The listing builds one solid part. Answer for the finished solid, in the listing's coordinates (mm). Round coordinates to 2 decimals unless told otherwise and drop trailing zeros. Write each loop counter-clockwise with the first axis right and the second up, starting at its lowest first coordinate (ties: lowest second). Pieces come first, ordered by that corner, then holes.
(1) Find the intervals of material crossed by probe 1 along Z at (x, y) = (25, 0.9); probe 2 along X at (y, z) = (1.8, -12.7); probe 3 along X at (y, z) = (0.45, -62), in increasing order.
(2) A cutting plane is placed at A-A, the plane z = -88.9. Give the vertices of the cut face in (x, y) (3 decimals).
(3) A cutting plane is placed at B-B, the plane y = 1.3. Give the number of separate pieces and of enclosed holes in the cut face, and give its area (3 significant figures).
(4) A cutting plane is placed at C-C, the plane z = -38. Give the vertices of the cut face in (x, y) (3 decimals).
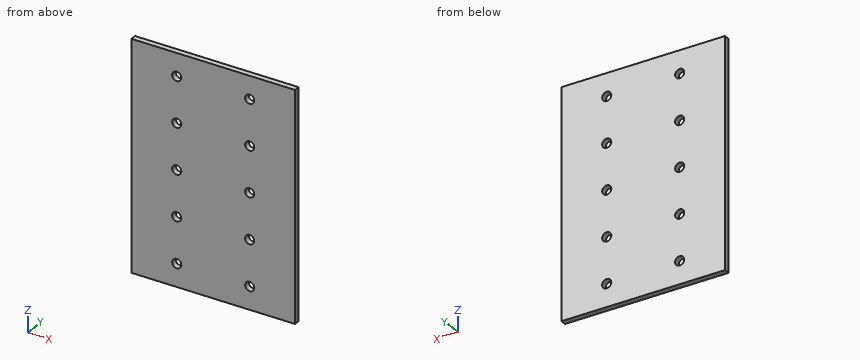
from build123d import *

# Parameters (mm, degrees)
SKETCH1_W           = 91.694
SKETCH1_H           = 127
BOSS_EXTRUDE1_DEPTH = 3.175
SKETCH2_R           = 2.5527
CUT_EXTRUDE1_DEPTH  = 3.175
LPATTERN1_COUNT     = 5
LPATTERN1_PITCH     = 25.4
SKETCH3_R           = 2.5527
CUT_EXTRUDE2_DEPTH  = 3.175
LPATTERN2_COUNT     = 5
LPATTERN2_PITCH     = 25.4


with BuildPart() as part:
    # Sketch1 → Boss-Extrude1 (new body)
    with BuildSketch(Plane(origin=(0, 0, 0), x_dir=(1, 0, 0), z_dir=(0, 1, 0))):
        with Locations((45.847, 63.5)):
            Rectangle(SKETCH1_W, SKETCH1_H)
    extrude(amount=BOSS_EXTRUDE1_DEPTH)

    # Sketch2 → Cut-Extrude1 (cut)
    with BuildSketch(Plane(origin=(0, 3.175, 0), x_dir=(1, 0, 0), z_dir=(0, 1, 0))):
        with Locations(Location((25.4, 12.7, 0), (0, 0, 270))):
            Circle(SKETCH2_R)
    cut_extrude1 = extrude(amount=-CUT_EXTRUDE1_DEPTH, mode=Mode.SUBTRACT)

    # LPattern1: Cut-Extrude1 ×5
    with Locations(*[(0, 0, -i * LPATTERN1_PITCH) for i in range(1, LPATTERN1_COUNT)]):
        add(cut_extrude1, mode=Mode.SUBTRACT)

    # Sketch3 → Cut-Extrude2 (cut)
    with BuildSketch(Plane(origin=(0, 3.175, 0), x_dir=(1, 0, 0), z_dir=(0, 1, 0))):
        with Locations(Location((66.294, 12.7, 0), (0, 0, 270))):
            Circle(SKETCH3_R)
    cut_extrude2 = extrude(amount=-CUT_EXTRUDE2_DEPTH, mode=Mode.SUBTRACT)

    # LPattern2: Cut-Extrude2 ×5
    with Locations(*[(0, 0, -i * LPATTERN2_PITCH) for i in range(1, LPATTERN2_COUNT)]):
        add(cut_extrude2, mode=Mode.SUBTRACT)


solid = part.part
Solutions:
1. probe 1: z = -127 to -116.82, -111.78 to -91.42, -86.38 to -66.02, -60.98 to -40.62, -35.58 to -15.22, -10.18 to 0
1. probe 2: x = 0 to 22.85, 27.95 to 63.74, 68.85 to 91.69
1. probe 3: x = 0 to 23.33, 27.47 to 64.23, 68.36 to 91.69
2. outline: (0, 0) - (22.847, 0) - (22.847, 3.175) - (0, 3.175) - close; (27.953, 0) - (63.741, 0) - (63.741, 3.175) - (27.953, 3.175) - close; (68.847, 0) - (91.694, 0) - (91.694, 3.175) - (68.847, 3.175) - close
3. separate pieces: 1
3. enclosed holes: 10
3. area: 11,400 mm2
4. outline: (0, 0) - (22.849, 0) - (22.849, 3.175) - (0, 3.175) - close; (27.951, 0) - (63.743, 0) - (63.743, 3.175) - (27.951, 3.175) - close; (68.845, 0) - (91.694, 0) - (91.694, 3.175) - (68.845, 3.175) - close
